Geometry check sheet. Reference: drawing and pictorial views, mm from the part's lowest x, y, z. A direction names the side the tool comes from. Give positions to 0.01 mm unless a question says otherwise; leave off trailing zeros. Write each loop counter-clockwise with the first axis right and the second up, starting at its lowest first coordinate (ties: lowest second). Pieces come first, ordered by that corner, then holes.
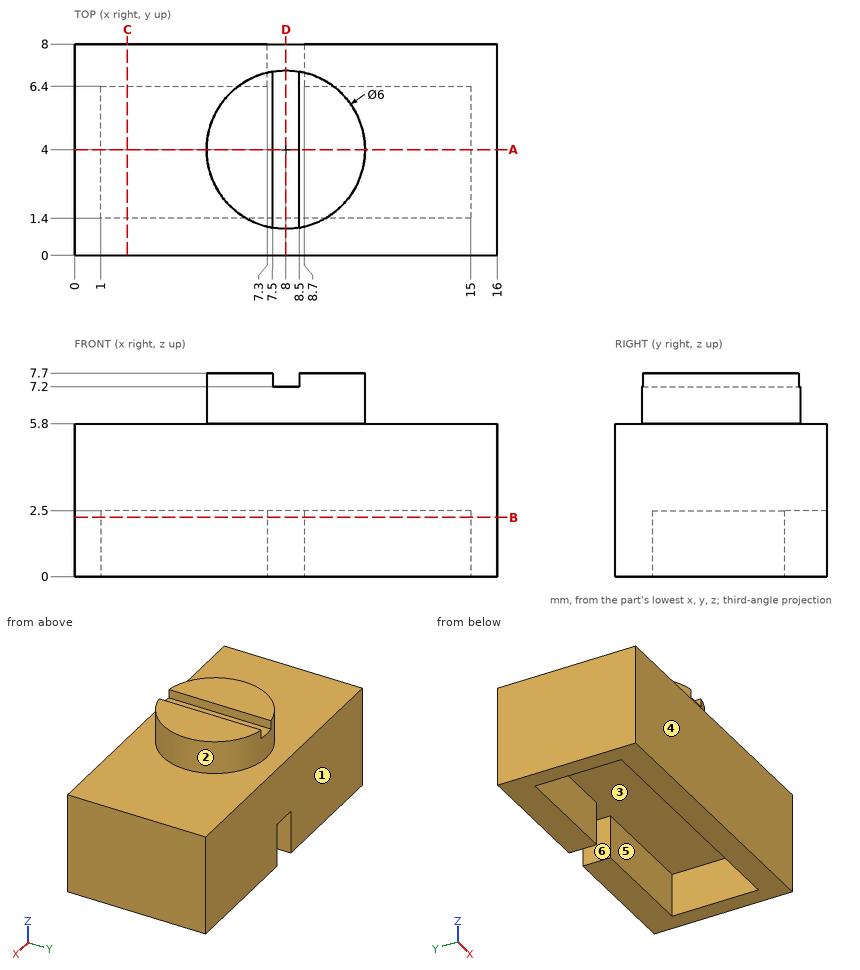
Item 1: Sectioned sample at C-C on x = 2. Record the cut outline in (y, z), then the cut area to 3 significant figures.
Answer key:
outline: (0, 0) - (1.4, 0) - (1.4, 2.5) - (6.4, 2.5) - (6.4, 0) - (8, 0) - (8, 5.8) - (0, 5.8) - close
area: 33.9 mm2
Item 2: Sectioned sample at B-B on z = 2.25. Record the cut outline in (x, y).
Answer key:
outline: (0, 0) - (16, 0) - (16, 8) - (8.7, 8) - (8.7, 6.4) - (15, 6.4) - (15, 1.4) - (1, 1.4) - (1, 6.4) - (7.3, 6.4) - (7.3, 8) - (0, 8) - close
Item 3: Depth check by flat-ended pin: pin 1 (1.5 mm diameter, centred on x = 5.5, y = 3.5, fed in from -Z). Enter the tip coordinate at first touch or a pass-through.
Answer key:
pin 1: stops at z = 2.5
Item 4: Sectioned sample at A-A on y = 4. Record the cut outline in (x, z), then the cut area to 3 significant figures.
Answer key:
outline: (0, 0) - (1, 0) - (1, 2.5) - (15, 2.5) - (15, 0) - (16, 0) - (16, 5.8) - (11, 5.8) - (11, 7.7) - (8.5, 7.7) - (8.5, 7.2) - (7.5, 7.2) - (7.5, 7.7) - (5, 7.7) - (5, 5.8) - (0, 5.8) - close
area: 68.7 mm2
Item 5: Release check for a two-part mould opening along X. For the marked faces 1, 2 and 3 record: released by +X, released by -X, zero draft, split by the parting line, or undercut.
Answer key:
face 1: zero draft
face 2: split by the parting line
face 3: undercut
Item 6: Scan lines: line 1 along Y through (x, z) = (7, 1); line 2 along X through (y, z) = (5, 0.5); line 3 along Z through (x, y) = (7.75, 3.5). Record each from-to range of solid material in increasing order.
Answer key:
line 1: y = 0 to 1.4, 6.4 to 8
line 2: x = 0 to 1, 15 to 16
line 3: z = 2.5 to 7.2
Item 7: Sectioned sample at D-D on x = 8. Record the cut outline in (y, z).
Answer key:
outline: (0, 0) - (1.4, 0) - (1.4, 2.5) - (8, 2.5) - (8, 5.8) - (7, 5.8) - (7, 7.2) - (1, 7.2) - (1, 5.8) - (0, 5.8) - close
Item 8: Set-up check for the marked faces 4, 5 and 6: record each of +Z, -Z, +X, -X, +Y, -Y from which the full face is reachable in a straight line by a thin tool's end or side.
Answer key:
face 4: +Z, -Z, +X, -X, -Y
face 5: -Z
face 6: -Z, +Y
